```python
from build123d import *

# Parameters (mm, degrees)
F1_DEPTH = 25
F3_DEPTH = 40


with BuildPart() as f1:
    # F0 (on Front) → F1 (new body)
    with BuildSketch(Plane.XZ):
        Polygon((0, 40), (0, 0), (50, 0), align=None)
    extrude(amount=F1_DEPTH)

    # F2 (on Top) → F3 (join)
    with BuildSketch(Plane.XY):
        Polygon((0, 45), (0, 0), (50, 0), (50, 20), (80, 20), (80, 45), align=None)
    extrude(amount=F3_DEPTH)


solid = f1.part
```
Work out the finished part from the listing and answer in its coordinate system (mm). A direction names the side the tool comes from. Give positions to 0.01 mm unless a question says otherwise; leave off trailing zeros. Write each loop counter-clockwise with the first axis right and the second up, starting at its lowest first coordinate (ties: lowest second). Pieces come first, ordered by that corner, then holes. Notation, with made-up numbers: (41, -24.5) -> (83, -24.5) arc R11 ccw to (83, -11.5) -> close; hole circle Ø3 at (37.25, -29). An arc over 180 degrees is marked (long way). Write item = value, one per line.
Q1. Section D-D on z = 16 is taken. Determine the outline of the cut face in (x, y), and give its area (3 significant figures).
Computed values:
outline = (0, -25) -> (30, -25) -> (30, 0) -> (50, 0) -> (50, 20) -> (80, 20) -> (80, 45) -> (0, 45) -> close
area = 3,750 mm^2
Q2. Flat-ended cylindrical pins translate along their axes: pin 1 Ø9 at (x, z) = (65, 24) entering from -Y; pin 2 Ø16 at (y, z) = (10.5, 19) entering from +X. Find the tip coordinate at first contact, or state that the pin passes through.
Computed values:
pin_1 = 20
pin_2 = 50
Q3. Section A-A on z = 6 is taken. Determine the outline of the cut face in (x, y), and give its area (3 significant figures).
Computed values:
outline = (0, -25) -> (42.5, -25) -> (42.5, 0) -> (50, 0) -> (50, 20) -> (80, 20) -> (80, 45) -> (0, 45) -> close
area = 4,060 mm^2
Q4. Section C-C on y = -10.5 is taken. Determine the outline of the cut face in (x, z).
Computed values:
outline = (0, 0) -> (50, 0) -> (0, 40) -> close
Q5. Consider line 1 along Y through (x, z) = (30.5, 30.5); line 2 along X through (y, z) = (6, 37); line 3 along Y through (x, z) = (60.5, 13). Determine where each line is inside the solid, lowest interval first.
Computed values:
line_1 = 0 to 45
line_2 = 0 to 50
line_3 = 20 to 45
Q6. Section B-B on x = 42 is taken. Determine the outline of the cut face in (y, z), and give its area (3 significant figures).
Computed values:
outline = (-25, 0) -> (45, 0) -> (45, 40) -> (0, 40) -> (0, 6.4) -> (-25, 6.4) -> close
area = 1,960 mm^2
Q7. A tool of negligible diameter and unlimited length cuts with its end or side. For faces 1 (the flat face through (65, 20, 20)), 2 (the flat face through (31, 10, 0)), 3 (the flat face through (25, -12, 20)), from which of +Z, -Z, +X, -X, +Y, -Y can it reach the whole face along a straight path? Write none if from no direction.
Computed values:
face_1 = +Z, -Z, +X, -Y
face_2 = -Z, +X, -X, +Y, -Y
face_3 = +Z, +X, -Y
